Check sheet for the drawn part. Datum: minimum x, y, z corner. Units: mm. A direction names the side the tool comes from. Coordinates: 2 decimals unless noted, no trailing zeros. Loops run counter-clockwise (first coordinate to the right, second up) from the corner with the lowest first, then second, coordinate; pieces in that order, holes last. Notation, with made-up numbers: M 61.5,-35 L 89.5,-35 A18 cw 89.5,-8 Z; hole C 47.25,-27.75 d3. An arc over 180 degrees is marked long. Answer in a Markdown table with one row per item. Add a question column.
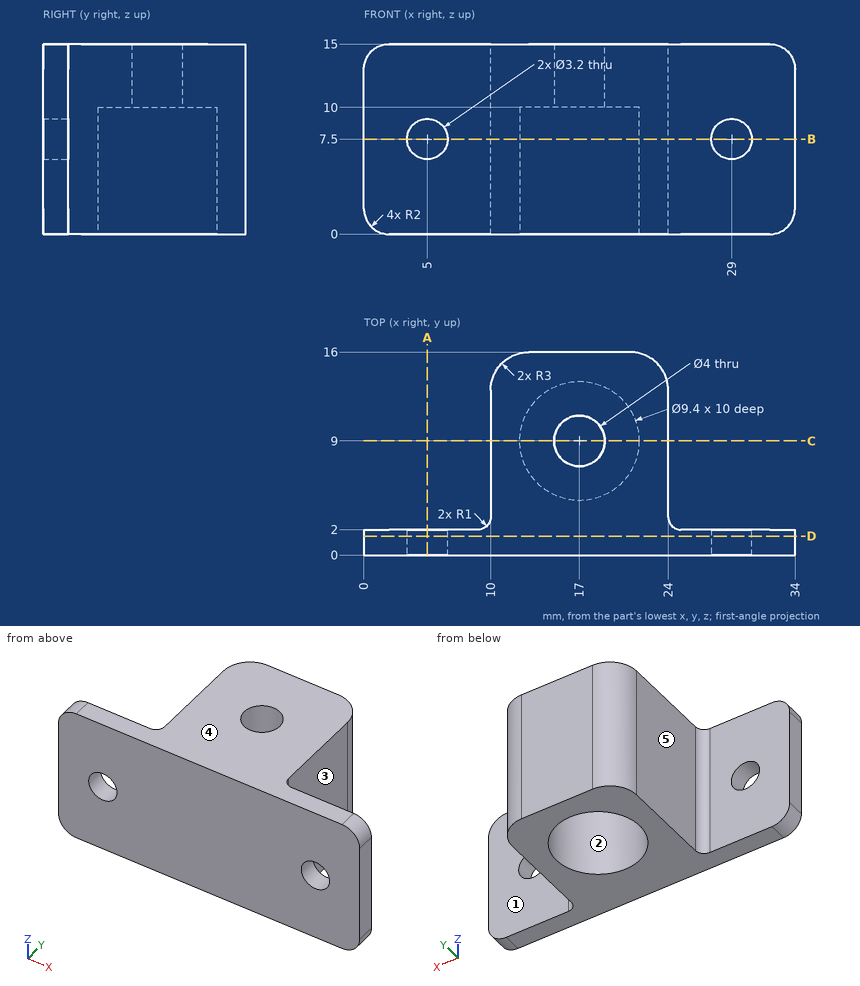
Q1. Mould release check, pull along Y, two halves, no side actions. Record for the marked faces 1, 2 and 3: released by +Y, released by -Y, zero draft, split by the parting line, or undercut.
Q2. Cross-section at A-A (x = 5). Record the cut outline in (y, z), plus the area to 3 significant figures.
Q3. Thickness scan on L1, parallel to Z at x = 29, y = 0.9; L2, parallel to X at y = 9, z = 6; L3, parallel to X at y = 9, z = 13.2. Record the ranges inside material, lowest first.
Q4. Cross-section at B-B (z = 7.5). Record the cut outline in (x, y), plus the area to 3 significant figures.
Q5. Cross-section at D-D (y = 1.5). Record the cut outline in (x, z), plus the area to 3 significant figures.
Q6. Cross-section at C-C (y = 9). Record the cut outline in (x, z).
Q7. Access from +Z, -Z, +X, -X, +Y, -Y to the whole of each face (thin tool, end or side, straight path). Record for the marked faces 4 and 5.
Q8. Go/stop test with flat-tipped pins: pin 1 (2.5 mm diameter, centred on x = 31.5, z = 5.5, fed in from +Y); pin 2 (5.5 mm diameter, centred on x = 17, y = 9, fed in from -Z); pin 3 (1 mm diameter, centred on y = 4, z = 6, fed in from +X). Record where each tip stops, or that it passes through.
Answer key:
| question | item | result |
|---|---|---|
| 1 | face 1 | released by +Y |
| 1 | face 2 | undercut |
| 1 | face 3 | zero draft |
| 2 | outline | M 0,0 L 2,0 L 2,5.9 L 0,5.9 Z; M 0,9.1 L 2,9.1 L 2,15 L 0,15 Z |
| 2 | area | 23.6 mm^2 |
| 3 | L1 | 0 to 5.9, 9.1 to 15 |
| 3 | L2 | 10 to 12.3, 21.7 to 24 |
| 3 | L3 | 10 to 15, 19 to 24 |
| 4 | outline | M 0,0 L 3.4,0 L 3.4,2 L 0,2 Z; M 6.6,0 L 27.4,0 L 27.4,2 L 25,2 A1 cw 24,3 L 24,13 A3 ccw 21,16 L 13,16 A3 ccw 10,13 L 10,3 A1 cw 9,2 L 6.6,2 Z; M 30.6,0 L 34,0 L 34,2 L 30.6,2 Z; hole C 17,9 d9.4 |
| 4 | area | 178 mm^2 |
| 5 | outline | M 0,2 A2 ccw 2,0 L 32,0 A2 ccw 34,2 L 34,13 A2 ccw 32,15 L 2,15 A2 ccw 0,13 Z; hole C 5,7.5 d3.2; hole C 29,7.5 d3.2 |
| 5 | area | 490 mm^2 |
| 6 | outline | M 10,0 L 12.3,0 L 12.3,10 L 15,10 L 15,15 L 10,15 Z; M 19,10 L 21.7,10 L 21.7,0 L 24,0 L 24,15 L 19,15 Z |
| 7 | face 4 | +Z, +X, -X, +Y, -Y |
| 7 | face 5 | +Z, -Z, -X, +Y |
| 8 | pin 1 | y = 2 |
| 8 | pin 2 | z = 10 |
| 8 | pin 3 | x = 24 |
